from build123d import *

# Parameters (mm, degrees)
F1_DEPTH = 60
F2_R     = 22.5
F3_DEPTH = 50
F4_R     = 1
F5_R     = 0.5


with BuildPart() as f1:
    # F0 (on Top) → F1 (new body)
    with BuildSketch(Plane.XY):
        Polygon((0, -50), (0, 0), (-3, 0), (-29.5, 0), (-29.5, -3), (-29.5, -35), (-26.5, -35), (-26.5, -3), (-3, -3), (-3, -47), (-53, -47), (-53, -50), (-48, -50), (-48, -110), (-45, -110), (-45, -50), (-8, -50), (-8, -110), (-5, -110), (-5, -50), (-3, -50), align=None)
    extrude(amount=F1_DEPTH)

    # F2 (on Right) → F3 (cut)
    with BuildSketch(Plane.YZ):
        with Locations((-94.5363938808, 30)):
            Circle(F2_R)
    extrude(amount=-F3_DEPTH, mode=Mode.SUBTRACT)

    # F4
    f4_edges = [f1.edges().sort_by_distance(p)[0] for p in [
        (-6.5, -110, 13.655983),
        (-6.5, -110, 46.344017),
        (-46.5, -110, 13.655983),
        (-46.5, -110, 46.344017),
        (-6.5, -110, 60),
        (-46.5, -110, 60),
        (-6.5, -110, 0),
        (-46.5, -110, 0),
    ]]
    fillet(f4_edges, radius=F4_R)

    # F5
    f5_edges = [f1.edges().sort_by_distance(p)[0] for p in [
        (-29.5, -35, 30),
        (-26.5, -35, 30),
        (-26.5, -19, 60),
        (-29.5, -17.5, 60),
        (-29.5, -17.5, 0),
        (-26.5, -19, 0),
        (-29.5, 0, 30),
        (-14.75, -3, 0),
        (-14.75, 0, 0),
        (-14.75, -3, 60),
        (-14.75, 0, 60),
        (0, 0, 30),
        (-26.5, -3, 30),
        (-3, -3, 30),
        (-3, -25, 60),
        (0, -25, 60),
        (-3, -25, 0),
        (0, -25, 0),
        (-28, -47, 60),
        (-26.5, -50, 60),
        (-50.5, -50, 60),
        (-2.5, -50, 60),
        (0, -50, 30),
        (-2.5, -50, 0),
        (-28, -47, 0),
        (-26.5, -50, 0),
        (-50.5, -50, 0),
        (-53, -47, 30),
        (-53, -50, 30),
    ]]
    fillet(f5_edges, radius=F5_R)


solid = f1.part
Verification items for the finished model (mm, model axes). A direction names the side the tool comes from. Round coordinates to 2 decimals unless told otherwise and drop trailing zeros. Loops run counter-clockwise (first coordinate to the right, second up) from the corner with the lowest first, then second, coordinate; pieces in that order, holes last. Notation, with made-up numbers: (66, 77) - (98, 77) arc R8 cw to (98, 89) - close; hole circle Ø5 at (-35.75, 78). An arc over 180 degrees is marked (long way). Use a Markdown table: item, result. Add a question column.
1. Section check B-B, the plane y = -16. Record the boundary of the cut face in (x, z), plus the area to 3 significant figures.
2. Release check for a two-part mould opening along Z. For faces 1 (the face through (-46.479, -72.047, 29.296)), 2 (the face through (-26.5, -19, 30)), 3 (the face through (-7, -50, 60)), 4 (the face through (-6.479, -72.047, 29.296)) record: released by +Z, released by -Z, zero draft, split by the parting line, or undercut.
3. Section check D-D, the plane x = -38. Record the boundary of the cut face in (y, z), plus the area to 3 significant figures.
4. Thickness scan on probe 1 along X at (y, z) = (-61, 23.5); probe 2 along Y at (x, z) = (-7.3, 30); probe 3 along Y at (x, z) = (-23, 14.5). Record the ranges inside material, lowest first. Write a range as [from, to].
5. Section check C-C, the plane y = -94. Record the boundary of the cut face in (x, z).
6. Section check A-A, the plane x = -19. Record the boundary of the cut face in (y, z).
7. Gauge pin test, flat ends, axial feed: pin 1 (12 mm diameter, centred on x = -36.5, z = 16, fed in from -Y); pin 2 (18 mm diameter, centred on y = -75, z = 31, fed in from +X); pin 3 (17 mm diameter, centred on y = -15.5, z = 44, fed in from -X). Record the tip position at first contact, or that the pin passes through.
8. Access from +Z, -Z, +X, -X, +Y, -Y to the whole of each face (thin tool, end or side, straight path). Record for faces 5 (the face through (-48, -66, 30)), 6 (the face through (-8, -66, 30)), 7 (the face through (-27, -47, 30)).
Checks:
| question | item | result |
|---|---|---|
| 1 | outline | (-29.5, 0.5) arc R0.5 ccw to (-29, 0) - (-27, 0) arc R0.5 ccw to (-26.5, 0.5) - (-26.5, 59.5) arc R0.5 ccw to (-27, 60) - (-29, 60) arc R0.5 ccw to (-29.5, 59.5) - close; (-3, 0.5) arc R0.5 ccw to (-2.5, 0) - (-0.5, 0) arc R0.5 ccw to (0, 0.5) - (0, 59.5) arc R0.5 ccw to (-0.5, 60) - (-2.5, 60) arc R0.5 ccw to (-3, 59.5) - close |
| 1 | area | 360 mm^2 |
| 2 | face 1 | undercut |
| 2 | face 2 | zero draft |
| 2 | face 3 | released by +Z |
| 2 | face 4 | undercut |
| 3 | outline | (-50, 0.5) arc R0.5 ccw to (-49.5, 0) - (-47.5, 0) arc R0.5 ccw to (-47, 0.5) - (-47, 59.5) arc R0.5 ccw to (-47.5, 60) - (-49.5, 60) arc R0.5 ccw to (-50, 59.5) - close |
| 3 | area | 180 mm^2 |
| 4 | probe 1 | x = [-48, -45], [-8, -5] |
| 4 | probe 2 | y = [-72.04, -47], [-3, 0] |
| 4 | probe 3 | y = [-50, -47], [-3, 0] |
| 5 | outline | (-48, 0) - (-45, 0) - (-45, 7.51) - (-48, 7.51) - close; (-48, 52.49) - (-45, 52.49) - (-45, 60) - (-48, 60) - close; (-8, 0) - (-5, 0) - (-5, 7.51) - (-8, 7.51) - close; (-8, 52.49) - (-5, 52.49) - (-5, 60) - (-8, 60) - close |
| 6 | outline | (-50, 0.5) arc R0.5 ccw to (-49.5, 0) - (-47.5, 0) arc R0.5 ccw to (-47, 0.5) - (-47, 59.5) arc R0.5 ccw to (-47.5, 60) - (-49.5, 60) arc R0.5 ccw to (-50, 59.5) - close; (-3, 0.5) arc R0.5 ccw to (-2.5, 0) - (-0.5, 0) arc R0.5 ccw to (0, 0.5) - (0, 59.5) arc R0.5 ccw to (-0.5, 60) - (-2.5, 60) arc R0.5 ccw to (-3, 59.5) - close |
| 7 | pin 1 | stops at y = -50 |
| 7 | pin 2 | stops at x = -5 |
| 7 | pin 3 | stops at x = -29.5 |
| 8 | face 5 | +Z, -Z, -X, -Y |
| 8 | face 6 | +Z, -Z, -Y |
| 8 | face 7 | +Z, -Z, -X |
